Verification items for this drawing (mm, ordinates from the low corner). A direction names the side the tool comes from. Coordinates: 2 decimals unless noted, no trailing zeros. Loops run counter-clockwise (first coordinate to the right, second up) from the corner with the lowest first, then second, coordinate; pieces in that order, holes last. Notation, with made-up numbers: M 62.5,-35 L 95.5,-35 A17 cw 95.5,-24 Z; hole C 34.25,30 d3. An arc over 180 degrees is marked long. One line per question, with ' | ' between items. Start each with the question number.
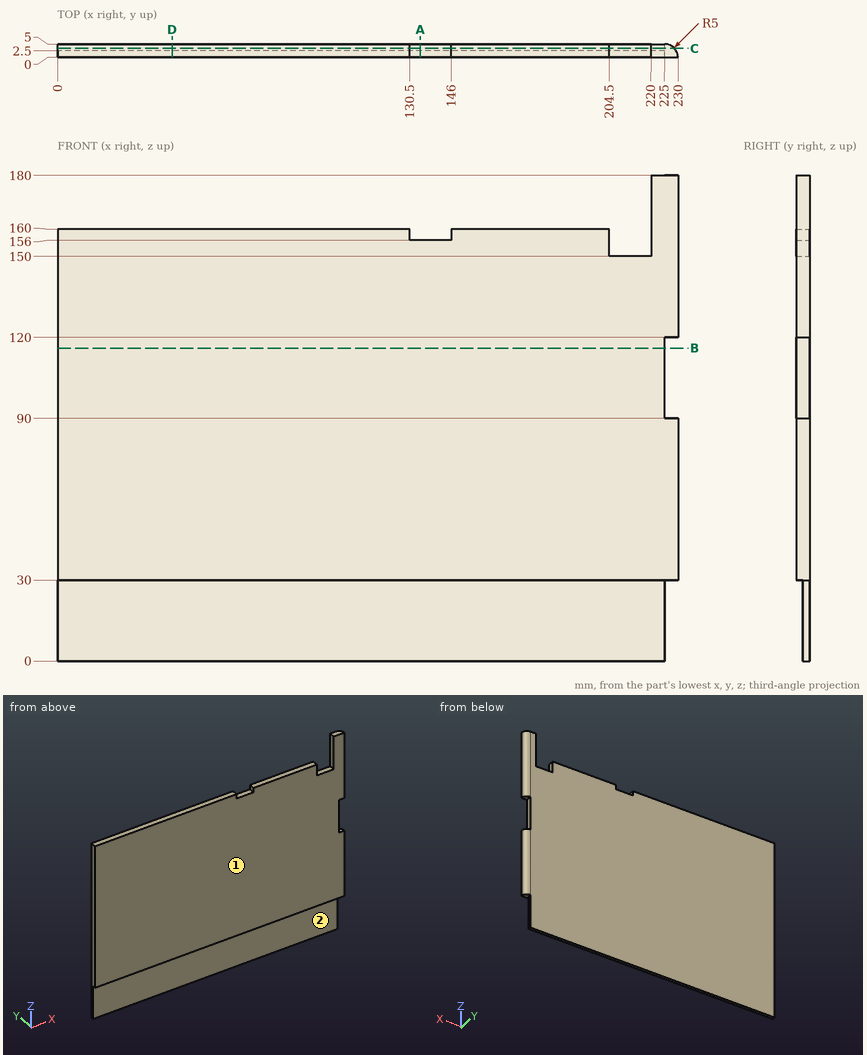
1. Depth check by flat-ended pin: pin 1 Ø2.5 at (x, y) = (39.5, 2) entering from +Z; pin 2 Ø1.5 at (y, z) = (2, 171.5) entering from -X; pin 3 Ø1.2 at (y, z) = (3, 12) entering from +X. Enter the tip coordinate at first touch or a pass-through.
2. Sectioned sample at D-D (x = 42.5). Record the cut outline in (y, z).
3. Thickness scan on line 1 (Z direction, x = 119.5, y = 4.25); line 2 (Z direction, x = 46, y = 1.6); line 3 (X direction, y = 4.8, z = 119.5). Record the ranges inside material, lowest first.
4. Sectioned sample at A-A (x = 134.5). Record the cut outline in (y, z), and give its area (3 significant figures).
5. Sectioned sample at B-B (z = 116). Record the cut outline in (x, y), and give its area (4 significant figures).
6. Tool access check on the marked faces 1 and 2. Record the directions out of +Z, -Z, +X, -X, +Y, -Y that give a thin tool (end or side, any length) a straight path to the whole face; none if there is none.
7. Sectioned sample at C-C (y = 3.4). Record the cut outline in (x, z).
Result:
1) pin 1: stops at z = 160 | pin 2: stops at x = 220 | pin 3: stops at x = 225
2) outline: M 0,30 L 2.5,30 L 2.5,0 L 5,0 L 5,160 L 0,160 Z
3) line 1: z = 0 to 160 | line 2: z = 30 to 160 | line 3: x = 0 to 225
4) outline: M 0,30 L 2.5,30 L 2.5,0 L 5,0 L 5,156 L 0,156 Z | area: 705 mm2
5) outline: M 0,0 L 225,0 L 225,5 L 0,5 Z | area: 1,125 mm2
6) face 1: +Z, -Z, +X, -X, -Y | face 2: -Z, +X, -X, -Y
7) outline: M 0,0 L 225,0 L 225,30 L 228.67,30 L 228.67,90 L 225,90 L 225,120 L 228.67,120 L 228.67,180 L 220,180 L 220,150 L 204.5,150 L 204.5,160 L 146,160 L 146,156 L 130.5,156 L 130.5,160 L 0,160 Z
